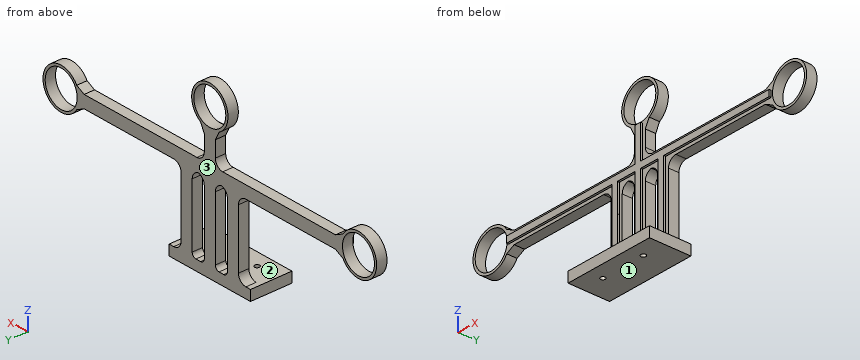
from build123d import *

# Parameters (mm, degrees)
SKETCH1_W           = 55.99938
SKETCH1_H           = 25.4
BOSS_EXTRUDE1_DEPTH = 6.35
BOSS_EXTRUDE2_DEPTH = 6.35
SKETCH10_R          = 10.999999971
CUT_EXTRUDE3_DEPTH  = 179.12779542
FILLET1_R           = 5.08
FILLET2_R           = 5.08
FILLET3_R           = 5.08
FILLET4_R           = 5.08
FILLET5_R           = 5.08
FILLET6_R           = 5.08
FILLET7_R           = 2.54
SKETCH9_R           = 1.5
CUT_EXTRUDE2_DEPTH  = 175.519471736
BOSS_EXTRUDE3_DEPTH = 1.27
FILLET8_R           = 1.27
CHAMFER1_SIZE       = 3.922074982
CHAMFER3_SIZE       = 3.922074982
CHAMFER4_SIZE       = 3.922074982


with BuildPart() as part:
    # Sketch1 → Boss-Extrude1 (new body)
    with BuildSketch(Plane.XY):
        with Locations((27.99969, -12.7)):
            Rectangle(SKETCH1_W, SKETCH1_H)
    extrude(amount=BOSS_EXTRUDE1_DEPTH)

    # Sketch2 → Boss-Extrude2 (add)
    with BuildSketch(Plane(origin=(0, 0, 0), x_dir=(1, 0, 0), z_dir=(0, 1, 0))):
        with BuildLine():
            ThreePointArc((118.420471835, -60.26605485), (142.825676579, -56.45605485), (118.420471835, -52.64605485))
            Line((118.420471835, -52.64605485), (47.74438, -52.64605485))
            Line((47.74438, -52.64605485), (47.74438, -6.35))
            Line((47.74438, -6.35), (40.124318317, -6.35))
            Line((40.124318317, -6.35), (40.124318317, -52.64605485))
            Line((40.124318317, -52.64605485), (31.80969, -52.64605485))
            Line((31.80969, -52.64605485), (31.80969, -6.35))
            Line((31.80969, -6.35), (24.18969, -6.35))
            Line((24.18969, -6.35), (24.18969, -52.64605485))
            Line((24.18969, -52.64605485), (15.882493554, -52.64605485))
            Line((15.882493554, -52.64605485), (15.882493554, -6.35))
            Line((15.882493554, -6.35), (8.262493554, -6.35))
            Line((8.262493554, -6.35), (8.262493554, -52.64605485))
            Line((8.262493554, -52.64605485), (-62.421091835, -52.64605485))
            ThreePointArc((-62.421091835, -52.64605485), (-86.826296579, -56.45605485), (-62.421091835, -60.26605485))
            Line((-62.421091835, -60.26605485), (24.18969, -60.26605485))
            Line((24.18969, -60.26605485), (24.18969, -78.963928031))
            ThreePointArc((24.18969, -78.963928031), (27.99969, -103.369132775), (31.80969, -78.963928031))
            Line((31.80969, -78.963928031), (31.80969, -60.26605485))
            Line((31.80969, -60.26605485), (118.420471835, -60.26605485))
        make_face()
    extrude(amount=-BOSS_EXTRUDE2_DEPTH)

    # Sketch10 → Cut-Extrude3 (cut, through all)
    with BuildSketch(Plane(origin=(0, 0, 0), x_dir=(1, 0, 0), z_dir=(0, 1, 0))):
        with Locations(Location((-74.326296579, -56.45605485, 0), (0, 0, 270))):
            Circle(SKETCH10_R)
        with Locations(Location((27.99969, -90.869132775, 0), (0, 0, 270))):
            Circle(SKETCH10_R)
        with Locations(Location((130.325676579, -56.45605485, 0), (0, 0, 270))):
            Circle(SKETCH10_R)
    extrude(amount=-CUT_EXTRUDE3_DEPTH, mode=Mode.SUBTRACT)

    # Fillet1
    fillet1_edges = [part.edges().sort_by_distance(p)[0] for p in [
        (8.262493554, -3.175, 6.35),
    ]]
    fillet(fillet1_edges, radius=FILLET1_R)

    # Fillet2
    fillet2_edges = [part.edges().sort_by_distance(p)[0] for p in [
        (47.74438, -3.175, 6.35),
    ]]
    fillet(fillet2_edges, radius=FILLET2_R)

    # Fillet3
    fillet3_edges = [part.edges().sort_by_distance(p)[0] for p in [
        (47.74438, -3.175, 52.64605485),
    ]]
    fillet(fillet3_edges, radius=FILLET3_R)

    # Fillet4
    fillet4_edges = [part.edges().sort_by_distance(p)[0] for p in [
        (8.262493554, -3.175, 52.64605485),
    ]]
    fillet(fillet4_edges, radius=FILLET4_R)

    # Fillet5
    fillet5_edges = [part.edges().sort_by_distance(p)[0] for p in [
        (31.80969, -3.175, 60.26605485),
        (24.18969, -3.175, 60.26605485),
    ]]
    fillet(fillet5_edges, radius=FILLET5_R)

    # Fillet6
    # the kernel refuses this fillet: 5.08 mm, written as the material it adds along each edge
    with BuildSketch(Plane(origin=(40.124318317, 0, 52.64605485), x_dir=(0, 0, -1), z_dir=(0, -1, 0)), Plane(origin=(24.18969, 0, 52.64605485), x_dir=(0, 0, -1), z_dir=(0, -1, 0))) as fillet6_piece_1:
        with BuildLine():
            CenterArc((FILLET6_R, -FILLET6_R), FILLET6_R, 90, 90)
            Line((0, -FILLET6_R), (0, 0))
            Line((0, 0), (FILLET6_R, 0))
        make_face()
    extrude(amount=6.35)
    with BuildSketch(Plane(origin=(31.80969, 0, 52.64605485), x_dir=(0, 0, -1), z_dir=(0, -1, 0)), Plane(origin=(15.882493554, 0, 52.64605485), x_dir=(0, 0, -1), z_dir=(0, -1, 0))) as fillet6_piece_2:
        with BuildLine():
            CenterArc((FILLET6_R, FILLET6_R), FILLET6_R, 180, 90)
            Line((0, FILLET6_R), (0, 0))
            Line((0, 0), (FILLET6_R, 0))
        make_face()
    extrude(amount=6.35)

    # Fillet7
    fillet7_edges = [part.edges().sort_by_distance(p)[0] for p in [
        (15.882493554, -3.175, 6.35),
        (24.18969, -3.175, 6.35),
        (31.80969, -3.175, 6.35),
        (40.124318317, -3.175, 6.35),
    ]]
    fillet(fillet7_edges, radius=FILLET7_R)

    # Sketch9 → Cut-Extrude2 (cut, through all)
    with BuildSketch(Plane.XY.offset(6.35)):
        with Locations((13.97, -16.51)):
            Circle(SKETCH9_R)
        with Locations((41.91, -16.51)):
            Circle(SKETCH9_R)
    extrude(amount=-CUT_EXTRUDE2_DEPTH, mode=Mode.SUBTRACT)

    # Sketch13 → Boss-Extrude3 (add)
    with BuildSketch(Plane.XZ.offset(6.35)):
        Polygon((-62.421091835, 58.361061908), (-62.421091835, 54.55105485), (10.160000409, 54.55105485), (10.160000409, 6.35), (13.97, 6.35), (13.946786012, 37.440717912), (13.946786012, 54.55105485), (26.09469, 54.55105485), (26.09469, 6.35), (29.90469, 6.35), (29.90469, 54.55105485), (42.02938, 54.55105485), (42.02938, 6.35), (45.83938, 6.35), (45.83938, 54.55105485), (118.420471835, 54.55105485), (118.420471835, 58.361061908), (29.90469, 58.361061908), (29.90469, 78.963928031), (26.09469, 78.963928031), (26.09469, 58.361061908), align=None)
    extrude(amount=BOSS_EXTRUDE3_DEPTH)

    # Fillet8
    fillet8_edges = [part.edges().sort_by_distance(p)[0] for p in [
        (10.160000409, -6.985, 6.35),
        (13.97, -6.985, 6.35),
        (42.02938, -6.985, 6.35),
        (45.83938, -6.985, 6.35),
        (26.09469, -6.985, 6.35),
        (29.90469, -6.985, 6.35),
    ]]
    fillet(fillet8_edges, radius=FILLET8_R)

    # Chamfer1
    # the kernel refuses this chamfer: 3.922074982, 2.54 mm, written as the material it adds along each edge
    with BuildSketch(Plane(origin=(-62.421091835, 0, 52.64605485), x_dir=(1, 0, 0), z_dir=(0, -1, 0))) as chamfer1_piece_1:
        with BuildLine():
            Line((CHAMFER1_SIZE, 0), (-1.195552336, -2.636188431))
            ThreePointArc((-1.195552336, -2.636188431), (-0.547031751, -1.409377958), (0, 0))
            Line((0, 0), (CHAMFER1_SIZE, 0))
        make_face()
    extrude(amount=6.35)
    with BuildSketch(Plane(origin=(-62.421091835, 0, 60.26605485), x_dir=(-0.4130254162108394, 0, 0.9107194988380687), z_dir=(0, -1, 0))) as chamfer1_piece_2:
        with BuildLine():
            Line((2.894621708, 0), (-CHAMFER1_SIZE * 0.413025416196, -CHAMFER1_SIZE * 0.910719498804))
            Line((-CHAMFER1_SIZE * 0.413025416196, -CHAMFER1_SIZE * 0.910719498804), (0, 0))
            ThreePointArc((0, 0), (1.509486004, -0.083916435), (2.894621708, 0))
        make_face()
    extrude(amount=6.35)

    # Chamfer3
    # the kernel refuses this chamfer: 3.922074982, 2.54 mm, written as the material it adds along each edge
    with BuildSketch(Plane(origin=(118.420471835, 0, 52.64605485), x_dir=(0.4130254162108416, 0, -0.9107194988380676), z_dir=(0, -1, 0))) as chamfer3_piece_1:
        with BuildLine():
            Line((2.894621708, 0), (-CHAMFER3_SIZE * 0.413025416196, -CHAMFER3_SIZE * 0.910719498804))
            Line((-CHAMFER3_SIZE * 0.413025416196, -CHAMFER3_SIZE * 0.910719498804), (0, 0))
            ThreePointArc((0, 0), (1.509486004, -0.083916435), (2.894621708, 0))
        make_face()
    extrude(amount=6.35)
    with BuildSketch(Plane(origin=(118.420471835, 0, 60.26605485), x_dir=(-1, 0, 0), z_dir=(0, -1, 0))) as chamfer3_piece_2:
        with BuildLine():
            Line((CHAMFER3_SIZE, 0), (-1.195552336, -2.636188431))
            ThreePointArc((-1.195552336, -2.636188431), (-0.547031751, -1.409377958), (0, 0))
            Line((0, 0), (CHAMFER3_SIZE, 0))
        make_face()
    extrude(amount=6.35)

    # Chamfer4
    # the kernel refuses this chamfer: 3.922074982, 2.54 mm, written as the material it adds along each edge
    with BuildSketch(Plane(origin=(31.80969, 0, 78.963928031), x_dir=(0.9107194988380676, 0, 0.4130254162108416), z_dir=(0, -1, 0))) as chamfer4_piece_1:
        with BuildLine():
            Line((2.894621708, 0), (-CHAMFER4_SIZE * 0.413025416196, -CHAMFER4_SIZE * 0.910719498804))
            Line((-CHAMFER4_SIZE * 0.413025416196, -CHAMFER4_SIZE * 0.910719498804), (0, 0))
            ThreePointArc((0, 0), (1.509486004, -0.083916435), (2.894621708, 0))
        make_face()
    extrude(amount=6.35)
    with BuildSketch(Plane(origin=(24.18969, 0, 78.963928031), x_dir=(0, 0, -1), z_dir=(0, -1, 0))) as chamfer4_piece_2:
        with BuildLine():
            Line((CHAMFER4_SIZE, 0), (-1.195552336, -2.636188431))
            ThreePointArc((-1.195552336, -2.636188431), (-0.547031751, -1.409377958), (0, 0))
            Line((0, 0), (CHAMFER4_SIZE, 0))
        make_face()
    extrude(amount=6.35)


solid = part.part
The listing builds one solid part. Answer for the finished solid, in the listing's coordinates (mm). Face numbers are marked on the shaded views. Round coordinates to 2 decimals unless told otherwise and drop trailing zeros. Loops run counter-clockwise (first coordinate to the right, second up) from the corner with the lowest first, then second, coordinate; pieces in that order, holes last. Notation, with made-up numbers: M 9.5,28.25 L 25.5,28.25 A30 ccw 25.5,54.25 Z; hole C 60,69 d11. An arc over 180 degrees is marked long. Return JSON: item names as keys, results as strings.
Q1. Find section C-C, the plane z = 18. Determine the outline of the cut face in (x, y).
Results list:
{"outline": "M 8.26,-6.35 L 10.16,-6.35 L 10.16,-7.62 L 13.96,-7.62 L 13.96,-6.35 L 15.88,-6.35 L 15.88,0 L 8.26,0 Z; M 24.19,-6.35 L 26.09,-6.35 L 26.09,-7.62 L 29.9,-7.62 L 29.9,-6.35 L 31.81,-6.35 L 31.81,0 L 24.19,0 Z; M 40.12,-6.35 L 42.03,-6.35 L 42.03,-7.62 L 45.84,-7.62 L 45.84,-6.35 L 47.74,-6.35 L 47.74,0 L 40.12,0 Z"}
Q2. Find section B-B, the plane x = -37.5. Determine the outline of the cut face in (y, z), plus the area to 3 significant figures.
Results list:
{"outline": "M -7.62,54.55 L -6.35,54.55 L -6.35,52.65 L 0,52.65 L 0,60.27 L -6.35,60.27 L -6.35,58.36 L -7.62,58.36 Z", "area": "53.2 mm2"}
Q3. Find the intervals of material crossed by line 1 along X through (y, z) = (-7, 46.5); line 2 along X through (y, z) = (-6, 14.5); line 3 along Y through (x, z) = (13.97, 1.75), in increasing order. Write a range as from..to.
Results list:
{"line 1": "x = 10.16..13.95, 26.09..29.9, 42.03..45.84", "line 2": "x = 8.26..15.88, 24.19..31.81, 40.12..47.74", "line 3": "y = -25.4..-18.01, -15.01..0"}
Q4. Each of these flat-tipped pins is pushed along its axis until it touches: pin 1 Ø3 at (x, z) = (96, 56) entering from -Y; pin 2 Ø1.4 at (y, z) = (-7, 33) entering from +X; pin 3 Ø7 at (y, z) = (-2, 33) entering from -X. Where does it stop, or does it pass through?
Results list:
{"pin 1": "stops at y = -7.62", "pin 2": "stops at x = 47.74", "pin 3": "stops at x = 8.26"}
Q5. The mould has two halves that part along Z. Classify the marked faces 1, 2 and 3: released by +Z, released by -Z, zero draft, split by the parting line, or undercut.
Results list:
{"face 1": "released by -Z", "face 2": "undercut", "face 3": "zero draft"}
Q6. Find section A-A, the plane z = 92. Determine the outline of the cut face in (x, y).
Results list:
{"outline": "M 15.55,-6.35 L 17.06,-6.35 L 17.06,0 L 15.55,0 Z; M 38.94,-6.35 L 40.45,-6.35 L 40.45,0 L 38.94,0 Z"}
Q7. Find section D-D, the plane y = -20.75. Determine the outline of the cut face in (x, z).
Results list:
{"outline": "M 0,0 L 56,0 L 56,6.35 L 0,6.35 Z"}
